Autodesk Inventor part; units mm, degrees
ref_plane "YZ Plane" through (0, 0, 0) normal (1, 0, 0) x (0, 1, 0)
ref_plane "XZ Plane" through (0, 0, 0) normal (0, 1, 0) x (-1, 0, 0)
ref_plane "XY Plane" through (0, 0, 0) normal (0, 0, 1) x (1, 0, 0)
sketch "Sketch1" plane through (0, 0, 0) normal (0, 0, 1) x (1, 0, 0)
  line L0 (0, 0) -> (0, 1092.2)
  line L1 (0, 1092.2) -> (812.8, 1092.2)
  line L2 (812.8, 1092.2) -> (812.8, 0)
  line L3 (812.8, 0) -> (0, 0)
  dimension "d0" = 1092.2
  dimension "d1" = 812.8
extrude "Extrusion1" add sketch "Sketch1" along normal blind 2641.6
sketch "Sketch2" plane through (812.8, 0, 0) normal (1, 0, 0) x (0, 0, -1)
  line L0 (-2641.6, 1092.2) -> (-2641.6, 0)
  line L1 (-2641.6, 0) -> (-2463.8, 0)
  line L2 (0, 0) -> (-2641.6, 0)
  line L3 (-2463.8, 0) -> (-2463.8, 1073.15)
  line L4 (-2463.8, 1073.15) -> (-2641.6, 1073.15)
  line L5 (-2641.6, 1073.15) -> (-2641.6, 0)
  line L6 (0, 1092.2) -> (0, 0)
  line L7 (0, 0) -> (-177.8, 0)
  line L8 (-177.8, 0) -> (-177.8, 1073.15)
  line L9 (-177.8, 1073.15) -> (0, 1073.15)
  line L10 (0, 1073.15) -> (0, 0)
  dimension "d4" = 177.8
  dimension "d5" = 1073.15
  dimension "d6" = 177.8
  dimension "d7" = 1073.15
extrude "Extrusion2" cut sketch "Sketch2" against normal blind 2641.6
sketch "Sketch3" plane through (812.8, 0, 2463.8) normal (0, 0, 1) x (1, 0, 0)
  line L0 (0, 0) -> (-812.8, 0)
  line L1 (-812.8, 0) -> (-635, 0)
  line L2 (-635, 0) -> (-635, 1073.15)
  line L3 (-812.8, 1073.15) -> (0, 1073.15)
  line L4 (-812.8, 1073.15) -> (-812.8, 0)
  line L5 (-812.8, 1092.2) -> (-812.8, 1073.15)
  line L6 (-635, 1073.15) -> (-812.8, 1073.15)
  dimension "d10" = 177.8
extrude "Extrusion3" cut sketch "Sketch3" against normal blind 2641.6
sketch "Sketch4" plane through (812.8, 0, 2463.8) normal (0, 0, 1) x (1, 0, 0)
  line L0 (0, 1073.15) -> (0, 0)
  line L1 (-635, 1073.15) -> (-635, 0)
  line L2 (-635, 0) -> (0, 0)
  line L3 (-635, 0) -> (-596.9, 0)
  line L4 (-596.9, 0) -> (-596.9, 19.05)
  line L5 (-596.9, 19.05) -> (-635, 19.05)
  line L6 (0, 0) -> (0, 1073.15)
  line L7 (0, 0) -> (0, 19.05)
  line L8 (0, 0) -> (-596.9, 0)
  line L9 (-596.9, 19.05) -> (-596.9, 1073.15)
  line L10 (-812.8, 1073.15) -> (0, 1073.15)
  line L11 (-635, 1073.15) -> (-596.9, 1073.15)
  line L12 (-635, 1073.15) -> (-635, 19.05)
  line L13 (-596.9, 19.05) -> (-558.8, 19.05)
  line L14 (-558.8, 19.05) -> (-558.8, 857.25)
  line L15 (-558.8, 857.25) -> (-596.9, 857.25)
  line L16 (-635, 0) -> (-635, 19.05)
  line L17 (-635, 19.05) -> (-25.4, 19.05)
  line L18 (-25.4, 19.05) -> (-25.4, 0)
  line L19 (-635, 0) -> (-25.4, 0)
  line L20 (-25.4, 19.05) -> (-63.5, 19.05)
  line L21 (-63.5, 19.05) -> (-63.5, 857.25)
  line L22 (-63.5, 857.25) -> (-25.4, 857.25)
  line L23 (-25.4, 857.25) -> (-25.4, 19.05)
  line L24 (-596.9, 857.25) -> (-596.9, 876.3)
  line L25 (-596.9, 876.3) -> (-25.4, 876.3)
  line L26 (-25.4, 876.3) -> (-25.4, 857.25)
  line L27 (-25.4, 857.25) -> (-596.9, 857.25)
  line L28 (-596.9, 876.3) -> (-596.9, 1092.2)
  line L29 (0, 1092.2) -> (-812.8, 1092.2)
  line L30 (-596.9, 1092.2) -> (0, 1092.2)
  line L31 (0, 1092.2) -> (0, 876.3)
  line L32 (-596.9, 876.3) -> (0, 876.3)
  line L33 (0, 876.3) -> (-25.4, 876.3)
  line L34 (-25.4, 876.3) -> (-25.4, 0)
  line L35 (0, 0) -> (-25.4, 0)
  line L36 (0, 0) -> (0, 876.3)
  point P0 (-812.8, 0)
  point P1 (-63.5, 857.25)
  point P2 (-25.4, 0)
  dimension "d13" = 635
  dimension "d15" = 19.05
  dimension "d16" = 38.1
  dimension "d17" = 838.2
  dimension "d18" = 609.6
  dimension "d19" = 38.1
  dimension "d20" = 838.2
  dimension "d21" = 19.05
extrude "Extrusion4" cut sketch "Sketch4" against normal blind 2641.6 contours L0 L32 L25 L9 L10 | L0 L2 L18 L23 L26 L32 | L21 L17 L14 L27
sketch "Sketch6" plane through (0, 1092.2, 0) normal (0, 1, 0) x (1, 0, 0)
  line L0 (0, 0) -> (0, -2641.6)
  line L1 (0, 0) -> (0, -177.8)
  line L2 (177.8, -2463.8) -> (177.8, -177.8)
  line L3 (0, -177.8) -> (177.8, -177.8)
  line L4 (177.8, -177.8) -> (355.6, -177.8)
  line L5 (177.8, -177.8) -> (787.4, -177.8)
  line L6 (177.8, -177.8) -> (177.8, 0)
  line L7 (812.8, 0) -> (0, 0)
  line L8 (177.8, 0) -> (812.8, 0)
  line L9 (812.8, -2641.6) -> (812.8, 0)
  line L10 (812.8, 0) -> (812.8, -355.6)
  line L11 (812.8, -355.6) -> (355.6, -355.6)
  line L12 (812.8, -2641.6) -> (812.8, -2286)
  line L13 (812.8, -2286) -> (355.6, -2286)
  line L14 (355.6, -2286) -> (355.6, -355.6)
  line L15 (812.8, -355.6) -> (812.8, -2286)
  dimension "d25" = 177.8
  dimension "d26" = 177.8
  dimension "d27" = 355.6
  dimension "d28" = 457.2
  dimension "d29" = 355.6
extrude "Extrusion5" cut sketch "Sketch6" against normal blind 25.4 contours L9 L13 L14 L11
sketch "Sketch7" plane through (215.9, 876.3, 2463.8) normal (0, 1, 0) x (1, 0, 0)
  line L0 (571.5, 0) -> (571.5, 2286)
  line L1 (0, 2286) -> (571.5, 2286)
  line L2 (571.5, 2286) -> (571.5, 2247.9)
  line L3 (0, 0) -> (0, 2286)
  line L4 (0, 2286) -> (0, 2247.9)
  line L5 (0, 2247.9) -> (571.5, 2247.9)
  line L6 (0, 0) -> (0, 38.1)
  line L7 (0, 38.1) -> (571.5, 38.1)
  line L8 (571.5, 0) -> (571.5, 38.1)
  line L9 (571.5, 0) -> (0, 0)
  point P0 (-215.9, 2463.8)
  point P1 (0, 38.1)
  dimension "d32" = 38.1
  dimension "d33" = 38.1
  dimension "d34" = 38.1
extrude "Extrusion6" add sketch "Sketch7" along normal blind 203.2 contours L9 L3 L7 L0 | L5 L3 L1 L0
sketch "Sketch8" plane through (177.8, 0, 177.8) normal (0, -1, 0) x (1, 0, 0)
  line L0 (609.6, 0) -> (609.6, 2286)
  line L1 (0, 2286) -> (0, 0)
  point P0 (-177.8, -177.8)
sketch "Sketch9" plane through (787.4, 0, 2463.8) normal (1, 0, 0) x (0, 0, -1)
  line L0 (38.1, 876.3) -> (2247.9, 876.3)
  line L1 (38.1, 876.3) -> (0, 876.3)
  line L2 (0, 1073.15) -> (0, 0)
  line L3 (0, 19.05) -> (0, 857.25)
  line L4 (0, 876.3) -> (0, 857.25)
  line L5 (0, 857.25) -> (2286, 857.25)
  line L6 (0, 857.25) -> (2286, 857.25)
  line L7 (2286, 857.25) -> (2286, 876.3)
  line L8 (2286, 0) -> (2286, 1073.15)
  line L9 (2286, 876.3) -> (0, 876.3)
  point P0 (2463.8, 0)
  dimension "d38" = 19.05
  dimension "d39" = 2286
extrude "Extrusion7" add sketch "Sketch9" along normal blind 25.4
sketch "Sketch10" plane through (215.9, 876.3, 215.9) normal (0, 1, 0) x (1, 0, 0)
  line L0 (596.9, 38.1) -> (596.9, -2247.9)
  line L1 (0, -2209.8) -> (0, 0)
  point P0 (-215.9, 215.9)
sketch "Sketch11" plane through (215.9, 876.3, 215.9) normal (1, 0, 0) x (0, 0, -1)
  line L0 (-2209.8, 0) -> (-2209.8, 196.85)
  line L1 (-2247.9, 196.85) -> (38.1, 196.85)
  line L2 (0, 0) -> (0, 196.85)
  line L3 (0, 196.85) -> (-2209.8, 196.85)
  line L4 (-2209.8, 0) -> (0, 0)
  line L5 (-2209.8, 0) -> (0, 0)
  line L6 (0, 0) -> (0, 196.85)
  line L7 (0, 0) -> (0, 196.85)
  point P0 (215.9, -876.3)
sketch "Sketch12" plane through (787.4, 0, 2463.8) normal (1, 0, 0) x (0, 0, -1)
  line L0 (0, 0) -> (0, 857.25)
  line L1 (0, 857.25) -> (2286, 857.25)
  line L2 (0, 0) -> (0, 857.25)
  line L3 (0, 857.25) -> (2286, 857.25)
  line L4 (2286, 857.25) -> (2286, 0)
  line L5 (2286, 857.25) -> (2286, 0)
  line L6 (2286, 0) -> (0, 0)
  point P0 (2463.8, 0)
extrude "Extrusion8" add sketch "Sketch12" along normal blind 25.4
sketch "Sketch13" plane through (787.4, 876.3, 2463.8) normal (1, 0, 0) x (0, 0, -1)
  line L0 (38.1, 0) -> (38.1, 196.85)
  line L1 (0, 196.85) -> (38.1, 196.85)
  line L2 (38.1, 196.85) -> (38.1, 0)
  line L3 (38.1, 0) -> (0, 0)
  line L4 (0, 0) -> (0, 196.85)
  point P0 (2463.8, -876.3)
extrude "Extrusion9" add sketch "Sketch13" along normal blind 25.4
sketch "Sketch14" plane through (787.4, 876.3, 177.8) normal (1, 0, 0) x (0, 0, -1)
  line L0 (-38.1, 0) -> (-38.1, 196.85)
  line L1 (0, 196.85) -> (0, 0)
  line L2 (-38.1, 196.85) -> (0, 196.85)
  line L3 (0, 196.85) -> (0, 0)
  line L4 (0, 0) -> (-38.1, 0)
  line L5 (-38.1, 0) -> (-38.1, 196.85)
  point P0 (177.8, -876.3)
extrude "Extrusion10" add sketch "Sketch14" along normal blind 25.4
sketch "Sketch15" plane through (812.8, 0, 2463.8) normal (1, 0, 0) x (0, 0, -1)
  line L0 (38.1, 876.3) -> (2247.9, 876.3)
  line L1 (0, 857.25) -> (2286, 857.25)
  line L2 (38.1, 876.3) -> (0, 876.3)
  line L3 (0, 876.3) -> (0, 857.25)
  line L4 (0, 857.25) -> (2286, 857.25)
  line L5 (2286, 0) -> (2286, 1073.15)
  line L6 (2286, 857.25) -> (2286, 876.3)
  line L7 (0, 876.3) -> (2286, 876.3)
  point P0 (2463.8, 0)
extrude "Extrusion11" add sketch "Sketch15" along normal blind 25.4
sketch "Sketch16" plane through (215.9, 876.3, 215.9) normal (0, 1, 0) x (1, 0, 0)
  line L0 (0, -2209.8) -> (596.9, -2209.8)
  line L1 (0, -2209.8) -> (38.1, -2209.8)
  point P0 (-215.9, 215.9)
  dimension "d51" = 38.1
sketch "Sketch17" plane through (215.9, 876.3, 215.9) normal (0, 1, 0) x (1, 0, 0)
  line L0 (0, -2209.8) -> (0, 0)
  line L1 (0, -2209.8) -> (38.1, -2209.8)
  line L2 (38.1, -2247.9) -> (38.1, 38.1)
  line L3 (38.1, -2209.8) -> (38.1, 0)
  line L4 (596.9, 0) -> (0, 0)
  line L5 (0, 0) -> (38.1, 4.2904)
  line L6 (38.1, 0) -> (0, 0)
  line L7 (0, 0) -> (0, -2209.8)
  point P0 (-215.9, 215.9)
  dimension "d52" = 38.1
extrude "Extrusion12" cut sketch "Sketch17" against normal blind 19.05 contours L0 L4 L2 L1
sketch "Sketch18" plane through (812.8, 0, 177.8) normal (0, 0, -1) x (-1, 0, 0)
  line L0 (558.8, 857.25) -> (63.5, 857.25)
  line L1 (63.5, 857.25) -> (38.1, 857.25)
  line L2 (38.1, 857.25) -> (38.1, 19.05)
  line L3 (38.1, 19.05) -> (63.5, 19.05)
  line L4 (63.5, 19.05) -> (63.5, 857.25)
  line L5 (63.5, 19.05) -> (63.5, 857.25)
  point P0 (812.8, 0)
  dimension "d58" = 25.4
  dimension "d59" = 838.2
extrude "Extrusion13" cut sketch "Sketch18" against normal blind 3810
sketch "Sketch21" plane through (254, 19.05, 2463.8) normal (1, 0, 0) x (0, 0, -1)
  line L0 (0, 0) -> (88.9, 0)
  line L1 (88.9, 0) -> (88.9, 838.2)
  line L2 (38.1, 838.2) -> (2247.9, 838.2)
  line L3 (88.9, 838.2) -> (0, 838.2)
  line L4 (0, 838.2) -> (0, 0)
  line L5 (88.9, 0) -> (787.4, 0)
  line L6 (0, 0) -> (2286, 0)
  line L7 (787.4, 0) -> (787.4, 838.2)
  line L8 (787.4, 838.2) -> (876.3, 838.2)
  line L9 (876.3, 838.2) -> (876.3, 0)
  line L10 (88.9, 838.2) -> (787.4, 838.2)
  line L11 (38.1, 838.2) -> (2247.9, 838.2)
  line L12 (876.3, 0) -> (1460.5, 0)
  line L13 (1460.5, 0) -> (1460.5, 838.2)
  line L14 (1460.5, 838.2) -> (1549.4, 838.2)
  line L15 (1549.4, 838.2) -> (1549.4, 0)
  line L16 (1549.4, 0) -> (1460.5, 0)
  line L17 (2286, 838.2) -> (2286, 0)
  line L18 (2286, 0) -> (2197.1, 0)
  line L19 (2197.1, 0) -> (2197.1, 838.2)
  line L20 (2197.1, 838.2) -> (1549.4, 838.2)
  line L21 (2197.1, 0) -> (1549.4, 0)
  line L22 (0, -19.05) -> (2286, -19.05)
  point P0 (2463.8, -19.05)
  point P1 (876.3, 0)
  dimension "d72" = 88.9
  dimension "d73" = 698.5
  dimension "d74" = 838.2
  dimension "d75" = 88.9
  dimension "d76" = 584.2
  dimension "d77" = 838.2
  dimension "d78" = 88.9
  dimension "d79" = 838.2
  dimension "d80" = 88.9
  dimension "d81" = 838.2
extrude "Extrusion14" cut sketch "Sketch21" along normal through all both and the other way through all contours L1 L2 L7 L5 | L9 L2 L13 L6 | L15 L2 L19 L6
sketch "Sketch22" plane through (812.8, 0, 177.8) normal (0, 0, -1) x (-1, 0, 0)
  line L0 (0, 876.3) -> (558.8, 876.3)
  line L1 (0, 876.3) -> (38.1, 876.3)
  point P0 (812.8, 0)
  dimension "d84" = 38.1
properties part number "bardraft"
Geometry: final body of the model. Coordinates: model frame, mm. A direction names the side the tool comes from. Round coordinates to 2 decimals unless told otherwise and drop trailing zeros. Write each loop counter-clockwise with the first axis right and the second up, starting at its lowest first coordinate (ties: lowest second). Pieces come first, ordered by that corner, then holes. Notation, with made-up numbers: M 88.5,59 L 135.5,59 A14 cw 135.5,86 Z; hole C 18,6.5 d9. An arc over 180 degrees is marked long. Answer in a Markdown table with one row per item. Add a question column.
(1) Contact query for flat-ended pins moving along their axis: pin 1 (19 mm diameter, centred on x = 800.5, y = 620, fed in from -Z); pin 2 (12 mm diameter, centred on y = 900, z = 2114, fed in from +X); pin 3 (21 mm diameter, centred on y = 867, z = 1145.5, fed in from -X). Output: stop coordinate, or through.
(2) Reachability of faces 1 (the face through (254, 432, 959)), 2 (the face through (215, 432, 2374.9)), 3 (the face through (812.8, 1033, 2451)), 4 (the face through (491, 0, 1305)), 5 (the face through (503, 887, 177.8)) from +Z, -Z, +X, -X, +Y, -Y: full face, straight path, thin tool, end or side. Return the list, or none.
(3) Cut plane D-D, the plane y = 485.5. Give the number of separate pieces and of enclosed holes in the cut face, then the cut area to 3 significant figures.
(4) Draft query along X for faces 6 (the face through (177.8, 892, 1241)), 7 (the face through (774.7, 444, 2419)), 8 (the face through (215, 444, 1587.5)). Return one class per face: pulls with the +X half, pulls with the -X half, needs draft (parallel to the pull), parting line crosses it, or undercut.
(5) Cut plane A-A, the plane z = 858. Return the cut outline in (x, y), then the cut area to 3 significant figures.
(6) Cut plane C-C, the plane x = 289. Return the cut outline in (y, z).
(7) Cut plane B-B, the plane x = 697. Return the cut outline in (y, z).
(8) Ray query, L1, parallel to Y at x = 313.5, z = 644.5; L2, parallel to Z at x = 791.5, y = 731.5; L3, parallel to Y at x = 798, z = 2423.5. Return the intervals inside material, ascending.
Established:
| question | item | result |
|---|---|---|
| 1 | pin 1 | z = 177.8 |
| 1 | pin 2 | x = 215.9 |
| 1 | pin 3 | x = 177.8 |
| 2 | face 1 | +Z, -Z |
| 2 | face 2 | +X, -X |
| 2 | face 3 | +Z, -Z, +X, +Y |
| 2 | face 4 | +Z, -Z, +X, -X, -Y |
| 2 | face 5 | -Z, +X, -X, -Y |
| 3 | separate pieces | 8 |
| 3 | enclosed holes | 0 |
| 3 | area | 40,600 mm² |
| 4 | face 6 | pulls with the -X half |
| 4 | face 7 | undercut |
| 4 | face 8 | needs draft |
| 5 | outline | M 0,1073.15 L 177.8,1073.15 L 177.8,857.25 L 215.9,857.25 L 215.9,1073.15 L 355.6,1073.15 L 355.6,1092.2 L 0,1092.2 Z; M 177.8,0 L 812.8,0 L 812.8,19.05 L 177.8,19.05 Z; M 254,857.25 L 838.2,857.25 L 838.2,876.3 L 254,876.3 Z |
| 5 | area | 38,200 mm² |
| 6 | outline | M 0,177.8 L 19.05,177.8 L 19.05,2463.8 L 0,2463.8 Z; M 857.25,177.8 L 1073.15,177.8 L 1073.15,0 L 1092.2,0 L 1092.2,2641.6 L 1073.15,2641.6 L 1073.15,2463.8 L 857.25,2463.8 Z; hole M 876.3,215.9 L 1073.15,215.9 L 1073.15,2425.7 L 876.3,2425.7 Z |
| 7 | outline | M 0,177.8 L 19.05,177.8 L 19.05,2463.8 L 0,2463.8 Z; M 857.25,177.8 L 1073.15,177.8 L 1073.15,0 L 1092.2,0 L 1092.2,355.6 L 1073.15,355.6 L 1073.15,215.9 L 876.3,215.9 L 876.3,2425.7 L 1073.15,2425.7 L 1073.15,2286 L 1092.2,2286 L 1092.2,2641.6 L 1073.15,2641.6 L 1073.15,2463.8 L 857.25,2463.8 Z |
| 8 | L1 | 0 to 19.05, 857.25 to 876.3, 1073.15 to 1092.2 |
| 8 | L2 | 177.8 to 266.7, 914.4 to 1003.3, 1587.5 to 1676.4, 2374.9 to 2463.8 |
| 8 | L3 | 0 to 876.3, 1073.15 to 1092.2 |
